For this review, take the finished solid that the model builds, in its own axes (mm). Face numbers are marked on the shaded views. A direction names the side the tool comes from. Give positions to 0.01 mm unless a question says otherwise; leave off trailing zeros. Order: outer loops, then holes, each group sorted by start corner. A loop starts at its lowest first (then second) coordinate and runs counter-clockwise, first axis right, second up. Notation, with made-up numbers: (-24.5, -31) - (3.5, -31) arc R26 ccw to (3.5, -17) - close; hole circle Ø6 at (34, 15.5). An arc over 180 degrees is marked (long way). Put each result on its own line as item: value. Start each with the question number.
```python
from build123d import *

# Parameters (mm, degrees)
F0_W     = 50.8
F0_H     = 50.8
F1_DEPTH = 12.7
F2_W     = 12.7
F2_H     = 50.8
F3_DEPTH = 25.4
F4_R     = 6.35
F5_DEPTH = 12.701


with BuildPart() as f1:
    # F0 (on Top) → F1 (new body)
    with BuildSketch(Plane.XY):
        with Locations((-35.357555, -12.31235)):
            Rectangle(F0_W, F0_H)
    extrude(amount=F1_DEPTH)

    # F2 (on face) → F3 (join)
    with BuildSketch(Plane.XY.offset(12.7)):
        with Locations((-16.307555, -12.31235)):
            Rectangle(F2_W, F2_H)
    extrude(amount=F3_DEPTH)

    # F4 (on face) → F5 (cut, through all)
    with BuildSketch(Plane(origin=(-22.657555, 0, 0), x_dir=(0, -1, 0), z_dir=(-1, 0, 0))):
        with Locations((12.31235, 25.4)):
            Circle(F4_R)
    extrude(amount=-F5_DEPTH, mode=Mode.SUBTRACT)


solid = f1.part
```
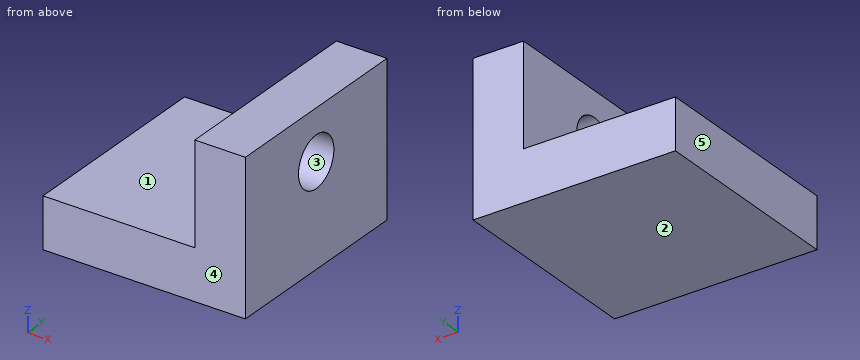
1. Add section D-D, the plane y = 3.5. Give the boundary of the cut face in (x, z).
2. Add section C-C, the plane x = -13.5. Give the boundary of the cut face in (y, z), then the cut area to 3 significant figures.
3. The part is to be moulded in two halves that separate along Y. For the marked faces 3, 4 and 5, say which applies: released by +Y, released by -Y, zero draft, split by the parting line, or undercut.
4. Tool access review of the marked faces 1 and 2: name each direction out of +Z, -Z, +X, -X, +Y, -Y from which nothing blocks a thin tool from reaching the whole face with its end or side.
5. Add section A-A, the plane z = 25.4. Give the boundary of the cut face in (x, y).
6. Wall thickness on line 1 (Y direction, x = -20, z = 25); line 2 (X direction, y = -19.5, z = 18.5); line 3 (Z direction, x = -39.5, y = 9): over which ranges is each line inside the solid? List them lowest first. Write a range as from..to.
7. Clearance check with flat-ended pins moving along their axes: pin 1 (11.5 mm diameter, centred on x = -46, y = -10, fed in from +Z); pin 2 (2 mm diameter, centred on y = -1, z = 18, fed in from -X). State where each tip first meets the part, or that it passes through.
8. Add section B-B, the plane y = -8. Give the boundary of the cut face in (x, z).
Found:
1. outline: (-60.76, 0) - (-9.96, 0) - (-9.96, 38.1) - (-22.66, 38.1) - (-22.66, 12.7) - (-60.76, 12.7) - close
2. outline: (-37.71, 0) - (13.09, 0) - (13.09, 38.1) - (-37.71, 38.1) - close; hole circle Ø12.7 at (-12.31, 25.4)
2. area: 1,810 mm^2
3. face 3: undercut
3. face 4: released by -Y
3. face 5: zero draft
4. face 1: +Z, -X, +Y, -Y
4. face 2: -Z, +X, -X, +Y, -Y
5. outline: (-22.66, -37.71) - (-9.96, -37.71) - (-9.96, -18.66) - (-22.66, -18.66) - close; (-22.66, -5.96) - (-9.96, -5.96) - (-9.96, 13.09) - (-22.66, 13.09) - close
6. line 1: y = -37.71..-18.65, -5.97..13.09
6. line 2: x = -22.66..-9.96
6. line 3: z = 0..12.7
7. pin 1: stops at z = 12.7
7. pin 2: stops at x = -22.66
8. outline: (-60.76, 0) - (-9.96, 0) - (-9.96, 20.74) - (-22.66, 20.74) - (-22.66, 12.7) - (-60.76, 12.7) - close; (-22.66, 30.06) - (-9.96, 30.06) - (-9.96, 38.1) - (-22.66, 38.1) - close
